```python
from build123d import *

# Parameters (mm, degrees)
SKETCH_1_R          = 1.05
EXTRUDE_1_DEPTH     = 2
SKETCH_2_R          = 3
CUT_EXTRUDE_1_DEPTH = 2
OTHER_1_OUTLINE_R   = 3
OTHER_1_DEPTH       = 2
FILLET_1_R          = 4


# Read off the part's stored shape, not the designer's step: 填充阵列1
with BuildPart() as part:
    # 草图1 → 凸台-拉伸1 (new body)
    with BuildSketch(Plane(origin=(0, 0, 0), x_dir=(1, 0, 0), z_dir=(0, 1, 0))):
        Polygon((110, 35), (110, 64), (0, 64), (0, 35), (-4, 35), (-4, 29), (0, 29), (0, 0), (110, 0), (110, 29), (114, 29), (114, 35), align=None)
        with Locations(Location((-1, 32, 0), (0, 0, 270))):
            Circle(SKETCH_1_R, mode=Mode.SUBTRACT)
        with Locations(Location((111, 32, 0), (0, 0, 270))):
            Circle(SKETCH_1_R, mode=Mode.SUBTRACT)
    extrude(amount=EXTRUDE_1_DEPTH)

    # 草图2 → 切除-拉伸1 (cut)
    with BuildSketch(Plane(origin=(0, 2, 0), x_dir=(1, 0, 0), z_dir=(0, 1, 0))):
        with Locations(Location((55, 33.05, 0), (0, 0, 270))):
            Circle(SKETCH_2_R)
    extrude(amount=-CUT_EXTRUDE_1_DEPTH, mode=Mode.SUBTRACT)

    # 填充阵列1 outline → 填充阵列1 (cut)
    with BuildSketch(Plane(origin=(0, 0, 0), x_dir=(1, 0, 0), z_dir=(0, 1, 0))):
        with Locations((10, 41.710254038)):
            Circle(OTHER_1_OUTLINE_R)
        with Locations((85, 33.05)):
            Circle(OTHER_1_OUTLINE_R)
        with Locations((90, 41.710254038)):
            Circle(OTHER_1_OUTLINE_R)
        with Locations((95, 50.370508076)):
            Circle(OTHER_1_OUTLINE_R)
        with Locations((85, 15.729491924)):
            Circle(OTHER_1_OUTLINE_R)
        with Locations((80, 24.389745962)):
            Circle(OTHER_1_OUTLINE_R)
        with Locations((75, 15.729491924)):
            Circle(OTHER_1_OUTLINE_R)
        with Locations((85, 50.370508076)):
            Circle(OTHER_1_OUTLINE_R)
        with Locations((80, 41.710254038)):
            Circle(OTHER_1_OUTLINE_R)
        with Locations((100, 24.389745962)):
            Circle(OTHER_1_OUTLINE_R)
        with Locations((90, 24.389745962)):
            Circle(OTHER_1_OUTLINE_R)
        with Locations((95, 33.05)):
            Circle(OTHER_1_OUTLINE_R)
        with Locations((100, 41.710254038)):
            Circle(OTHER_1_OUTLINE_R)
        with Locations((95, 15.729491924)):
            Circle(OTHER_1_OUTLINE_R)
        with Locations((30, 41.710254038)):
            Circle(OTHER_1_OUTLINE_R)
        with Locations((35, 50.370508076)):
            Circle(OTHER_1_OUTLINE_R)
        with Locations((25, 15.729491924)):
            Circle(OTHER_1_OUTLINE_R)
        with Locations((30, 24.389745962)):
            Circle(OTHER_1_OUTLINE_R)
        with Locations((35, 15.729491924)):
            Circle(OTHER_1_OUTLINE_R)
        with Locations((45, 50.370508076)):
            Circle(OTHER_1_OUTLINE_R)
        with Locations((40, 41.710254038)):
            Circle(OTHER_1_OUTLINE_R)
        with Locations((35, 33.05)):
            Circle(OTHER_1_OUTLINE_R)
        with Locations((20, 41.710254038)):
            Circle(OTHER_1_OUTLINE_R)
        with Locations((15, 33.05)):
            Circle(OTHER_1_OUTLINE_R)
        with Locations((10, 24.389745962)):
            Circle(OTHER_1_OUTLINE_R)
        with Locations((15, 50.370508076)):
            Circle(OTHER_1_OUTLINE_R)
        with Locations((25, 33.05)):
            Circle(OTHER_1_OUTLINE_R)
        with Locations((20, 24.389745962)):
            Circle(OTHER_1_OUTLINE_R)
        with Locations((15, 15.729491924)):
            Circle(OTHER_1_OUTLINE_R)
        with Locations((25, 50.370508076)):
            Circle(OTHER_1_OUTLINE_R)
        with Locations((55, 15.729491924)):
            Circle(OTHER_1_OUTLINE_R)
        with Locations((60, 24.389745962)):
            Circle(OTHER_1_OUTLINE_R)
        with Locations((65, 33.05)):
            Circle(OTHER_1_OUTLINE_R)
        with Locations((70, 41.710254038)):
            Circle(OTHER_1_OUTLINE_R)
        with Locations((75, 33.05)):
            Circle(OTHER_1_OUTLINE_R)
        with Locations((70, 24.389745962)):
            Circle(OTHER_1_OUTLINE_R)
        with Locations((65, 15.729491924)):
            Circle(OTHER_1_OUTLINE_R)
        with Locations((75, 50.370508076)):
            Circle(OTHER_1_OUTLINE_R)
        with Locations((40, 24.389745962)):
            Circle(OTHER_1_OUTLINE_R)
        with Locations((45, 33.05)):
            Circle(OTHER_1_OUTLINE_R)
        with Locations((50, 41.710254038)):
            Circle(OTHER_1_OUTLINE_R)
        with Locations((55, 50.370508076)):
            Circle(OTHER_1_OUTLINE_R)
        with Locations((45, 15.729491924)):
            Circle(OTHER_1_OUTLINE_R)
        with Locations((50, 24.389745962)):
            Circle(OTHER_1_OUTLINE_R)
        with Locations((60, 41.710254038)):
            Circle(OTHER_1_OUTLINE_R)
        with Locations((65, 50.370508076)):
            Circle(OTHER_1_OUTLINE_R)
    extrude(amount=OTHER_1_DEPTH, mode=Mode.SUBTRACT)

    # 圆角1
    fillet_1_edges = [part.edges().sort_by_distance(p)[0] for p in [
        (110, 1, -29),
        (110, 1, -35),
        (0, 1, -35),
        (0, 1, -29),
    ]]
    fillet(fillet_1_edges, radius=FILLET_1_R - 0.0001)  # a hair under: the kernel refuses the full size


solid = part.part
```
Source: CAD feature listing. Evaluate the final solid. Frame: model axes, mm. Give positions to 0.01 mm unless a question says otherwise; leave off trailing zeros. Loops run counter-clockwise (first coordinate to the right, second up) from the corner with the lowest first, then second, coordinate; pieces in that order, holes last. Notation, with made-up numbers: (57.25, 24.25) -> (116.25, 24.25) arc R11 ccw to (116.25, 30.25) -> close; hole circle Ø7 at (72, 39). An arc over 180 degrees is marked (long way). Use a Markdown table: item, result. Add a question column.
(1) Ray query, line 1 (Z direction, x = 65, y = 1.55); line 2 (Z direction, x = 100, y = 1.35); line 3 (Z direction, x = 42.5, y = 0.7). Return the intervals inside material, ascending.
(2) Section query A-A (x = 100). Output: boundary loops of the cut face in (y, z).
(3) First-contact query: pin 1 Ø5 at (x, z) = (25, -50.37) entering from -Y; pin 2 Ø1 at (y, z) = (0.5, -43.5) entering from -X. Flat tips, straight axial feed; report the tip coordinate or a pass-through.
(4) Section query B-B (x = 55). Output: boundary loops of the cut face in (y, z), then the cut area to 3 significant figures.
(5) Section query C-C (z = -22.5). Count the separate pieces of the cut face and the enclosed holes in it, then the cut area to 3 significant figures.
Checked values:
| question | item | result |
|---|---|---|
| 1 | line 1 | -64 to -53.37, -47.37 to -36.05, -30.05 to -18.73, -12.73 to 0 |
| 1 | line 2 | -64 to -44.71, -38.71 to -27.39, -21.39 to 0 |
| 1 | line 3 | -64 to -52.03, -48.71 to -43.37, -40.05 to -34.71, -31.39 to -26.05, -22.73 to -17.39, -14.07 to 0 |
| 2 | outline | (0, -64) -> (2, -64) -> (2, -44.71) -> (0, -44.71) -> close; (0, -38.71) -> (2, -38.71) -> (2, -27.39) -> (0, -27.39) -> close; (0, -21.39) -> (2, -21.39) -> (2, 0) -> (0, 0) -> close |
| 3 | pin 1 | through |
| 3 | pin 2 | x = 0 |
| 4 | outline | (0, -64) -> (2, -64) -> (2, -53.37) -> (0, -53.37) -> close; (0, -47.37) -> (2, -47.37) -> (2, -36.05) -> (0, -36.05) -> close; (0, -30.05) -> (2, -30.05) -> (2, -18.73) -> (0, -18.73) -> close; (0, -12.73) -> (2, -12.73) -> (2, 0) -> (0, 0) -> close |
| 4 | area | 92.0 mm^2 |
| 5 | separate pieces | 11 |
| 5 | enclosed holes | 0 |
| 5 | area | 127 mm^2 |
